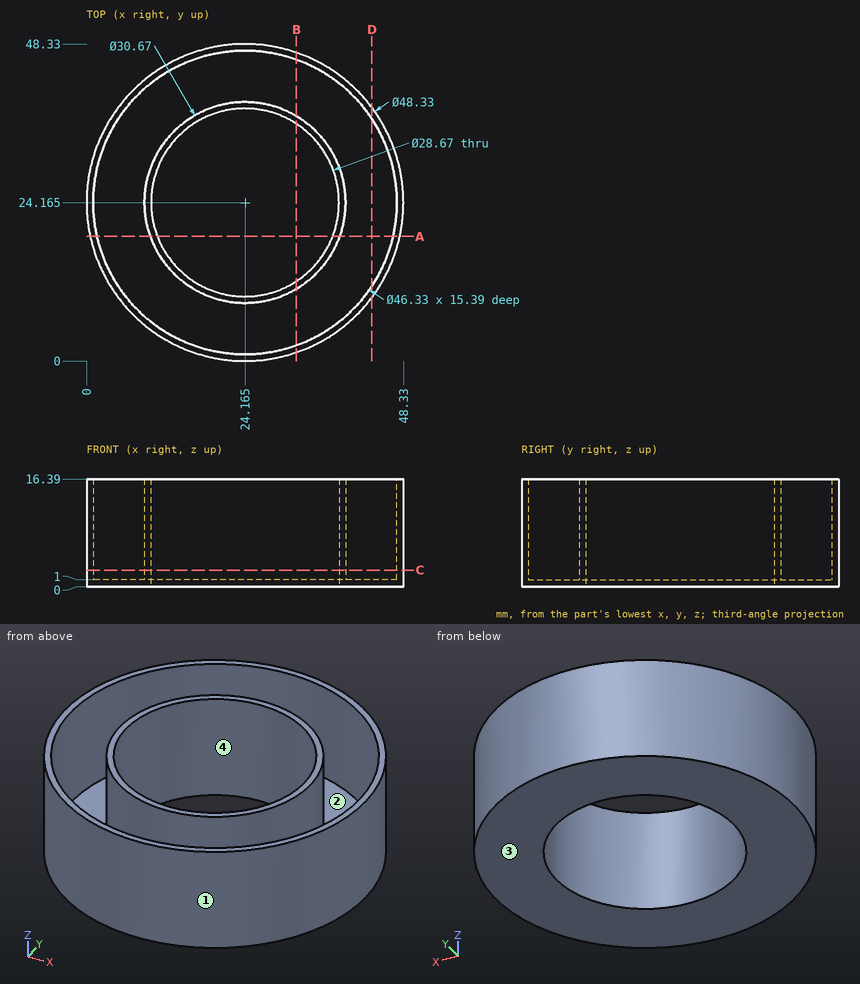
Job drawing, mm, ordinate dimensions from the low corner. One solid piece. Coordinates: 2 decimals unless noted, no trailing zeros. Order: outer loops, then holes, each group sorted by start corner. A loop starts at its lowest first (then second) coordinate and runs counter-clockwise, first axis right, second up. Notation, with made-up numbers: (85.5, 81.5) - (132.5, 81.5) arc R15 ccw to (132.5, 93.5) - close; hole circle Ø11 at (18.25, 2). An arc over 180 degrees is marked (long way). Write each question's results on one line, items separated by ' | '. Start each with the question number.
Item 1: Band-saw the part on B-B on x = 32. Write the cut outline in (y, z).
Item 2: Flat gauge pins, fed straight in: pin 1 (17 mm diameter, centred on x = 24.165, y = 24.165, fed in from -Z); pin 2 (8 mm diameter, centred on x = 13, z = 13, fed in from +Y); pin 3 (1 mm diameter, centred on x = 43, z = 10, fed in from +Y); pin 4 (2 mm diameter, centred on y = 42.5, z = 4, fed in from -X). Where does each tip first touch, or does it go through?
Item 3: Band-saw the part on C-C on z = 2.5. Write the cut outline in (x, y) (3 decimals).
Item 4: Band-saw the part on A-A on y = 19. Write the cut outline in (x, z), and give its area (3 significant figures).
Item 5: Band-saw the part on D-D on x = 43.5. Write the cut outline in (y, z).
Item 6: Mould opens along Y. For the marked faces 1, 2, 3 and 4 say: released by +Y, released by -Y, zero draft, split by the parting line, or undercut.
Item 7: Wall check: probe 1 along X at (y, z) = (17, 6.5); probe 2 along X at (y, z) = (19, 4.75); probe 3 along Y at (x, z) = (19.5, 11.5). Give the ranges that are in metal, low to high. Write a range as [from, to].
Numbers:
1) outline: (1.31, 0) - (12.16, 0) - (12.16, 16.39) - (10.98, 16.39) - (10.98, 1) - (2.37, 1) - (2.37, 16.39) - (1.31, 16.39) - close; (36.17, 0) - (47.02, 0) - (47.02, 16.39) - (45.96, 16.39) - (45.96, 1) - (37.35, 1) - (37.35, 16.39) - (36.17, 16.39) - close
2) pin 1: through | pin 2: y = 47.24 | pin 3: y = 39.91 | pin 4: x = 7.33
3) outline: circle Ø48.33 at (24.165, 24.165); circle Ø30.67 at (24.165, 24.165); hole circle Ø46.33 at (24.165, 24.165); hole circle Ø28.67 at (24.165, 24.165)
4) outline: (0.56, 0) - (10.79, 0) - (10.79, 16.39) - (9.73, 16.39) - (9.73, 1) - (1.58, 1) - (1.58, 16.39) - (0.56, 16.39) - close; (37.54, 0) - (47.77, 0) - (47.77, 16.39) - (46.75, 16.39) - (46.75, 1) - (38.6, 1) - (38.6, 16.39) - (37.54, 16.39) - close | area: 84.8 mm^2
5) outline: (9.67, 0) - (38.66, 0) - (38.66, 16.39) - (36.92, 16.39) - (36.92, 1) - (11.41, 1) - (11.41, 16.39) - (9.67, 16.39) - close
6) face 1: split by the parting line | face 2: undercut | face 3: zero draft | face 4: undercut
7) probe 1: [1.09, 2.14], [10.61, 11.75], [36.58, 37.72], [46.19, 47.24] | probe 2: [0.56, 1.58], [9.73, 10.79], [37.54, 38.6], [46.75, 47.77] | probe 3: [0.45, 1.47], [9.56, 10.61], [37.72, 38.77], [46.86, 47.88]
